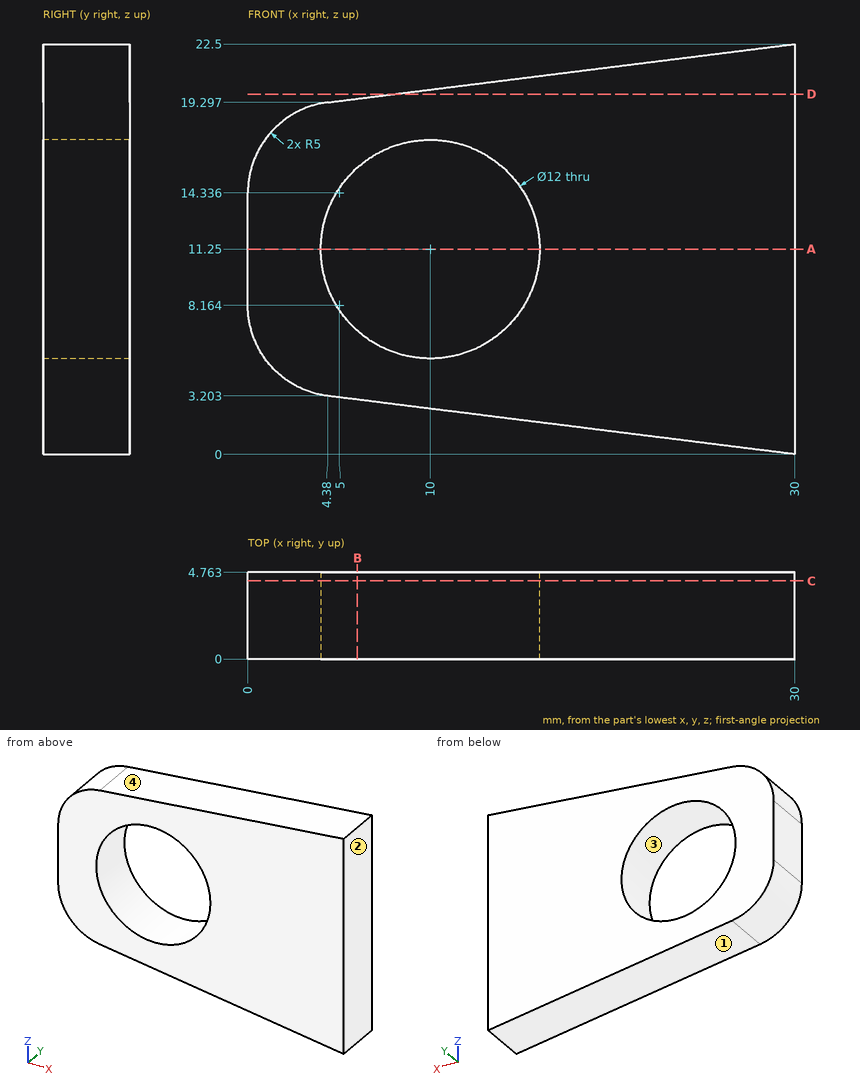
For this review, use the dimensioned drawing (mm, ordinates from the lowest corner) and the shaded views. Coordinates: 2 decimals unless noted, no trailing zeros. Order: outer loops, then holes, each group sorted by start corner. A loop starts at its lowest first (then second) coordinate and runs counter-clockwise, first axis right, second up. Notation, with made-up numbers: M 5,66 L 34,66 A25 ccw 34,95 Z; hole C 40.5,33.25 d3. An arc over 180 degrees is marked long. Answer as a JSON object with one key per item and string values. Group by question number.
1) Add section C-C, the plane y = 4.3. Write out the cut boundary in (x, z).
2) Add section B-B, the plane x = 6. Write out the cut boundary in (y, z).
3) For pin 1 (6 mm diameter, centred on x = 21.5, z = 9, fed in from -Y); pin 2 (1 mm diameter, centred on x = 25, y = 2.5, fed in from -Z), all flat-tipped, find the tip position at first contact; note any pin that passes through.
4) Add section A-A, the plane z = 11.25. Write out the cut boundary in (x, y).
5) Wall thickness on L1, parallel to X at y = 2.1, z = 11.25; L2, parallel to Z at x = 10, y = 1.65; L3, parallel to X at y = 3.45, z = 6 (1 decimal): over which ranges is each line inside the solid? List them lowest first.
6) Add section D-D, the plane z = 19.75. Write out the cut boundary in (x, y).
7) Mouldability with a two-part tool opening along Z and no side actions: class the marked faces 1, 2, 3 and 4 as pulls with the +Z half, pulls with the -Z half, needs draft (parallel to the pull), parting line crosses it, or undercut.
Computed values:
{
 "1": {"outline": "M 0,8.16 A5 ccw 4.38,3.2 L 30,0 L 30,22.5 L 4.38,19.3 A5 ccw 0,14.34 Z; hole C 10,11.25 d12"},
 "2": {"outline": "M 0,3 L 4.76,3 L 4.76,6.78 L 0,6.78 Z; M 0,15.72 L 4.76,15.72 L 4.76,19.5 L 0,19.5 Z"},
 "3": {"pin 1": "stops at y = 0", "pin 2": "stops at z = 0.56"},
 "4": {"outline": "M 0,0 L 4,0 L 4,4.76 L 0,4.76 Z; M 16,0 L 30,0 L 30,4.76 L 16,4.76 Z"},
 "5": {"L1": "x = 0 to 4, 16 to 30", "L2": "z = 2.5 to 5.25, 17.25 to 20", "L3": "x = 0.5 to 7.1, 12.9 to 30"},
 "6": {"outline": "M 8,0 L 30,0 L 30,4.76 L 8,4.76 Z"},
 "7": {"face 1": "pulls with the -Z half", "face 2": "needs draft", "face 3": "undercut", "face 4": "pulls with the +Z half"}
}
